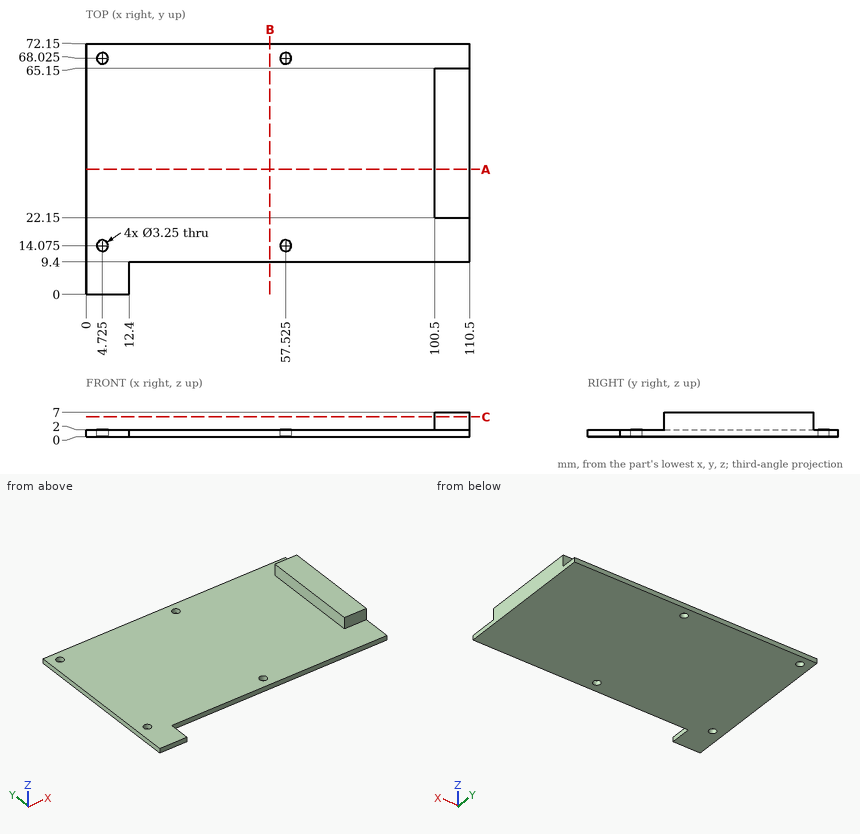
Study the drawing (mm; zero at the part's minimum x, y, z) and answer. Coordinates: 2 decimals unless noted, no trailing zeros. Write each loop counter-clockwise with the first axis right and the second up, starting at its lowest first coordinate (ties: lowest second). Pieces come first, ordered by that corner, then holes. Notation, with made-up numbers: (-18.5, 29.25) - (23.5, 29.25) arc R17 ccw to (23.5, 61.25) - close; hole circle Ø7 at (67, -9). An arc over 180 degrees is marked (long way). Return JSON: item names as keys, results as strings. Group by question number.
1. Given pin 1 (3 mm diameter, centred on x = 4.725, y = 68.025, fed in from -Z); pin 2 (4 mm diameter, centred on y = 49.5, z = 5.5, fed in from -X); pin 3 (0.6 mm diameter, centred on x = 60.5, z = 0.5, fed in from -Y); pin 4 (2.5 mm diameter, centred on x = 106.5, z = 4.5, fed in from +Y), each flat-ended and moving along its own axis, determine where each tip first touches the part or whether it passes through.
2. Straight lines are drawn through the part: L1, parallel to Z at x = 93, y = 48.5; L2, parallel to X at y = 55, z = 4; L3, parallel to Y at x = 97.5, z = 1.75. For each, find the intervals that lie inside material, in ascending order.
3. A cutting plane is placed at A-A, the plane y = 36. Determine the outline of the cut face in (x, z), plus the area to 3 significant figures.
4. A cutting plane is placed at B-B, the plane x = 53. Determine the outline of the cut face in (y, z), plus the area to 4 significant figures.
5. A cutting plane is placed at C-C, the plane z = 5.75. Determine the outline of the cut face in (x, y).
Ans:
{
 "1": {"pin 1": "through", "pin 2": "x = 100.5", "pin 3": "y = 9.4", "pin 4": "y = 65.15"},
 "2": {"L1": "0 to 2", "L2": "100.5 to 110.5", "L3": "9.4 to 72.15"},
 "3": {"outline": "(0, 0) - (110.5, 0) - (110.5, 7) - (100.5, 7) - (100.5, 2) - (0, 2) - close", "area": "271 mm²"},
 "4": {"outline": "(9.4, 0) - (72.15, 0) - (72.15, 2) - (9.4, 2) - close", "area": "125.5 mm²"},
 "5": {"outline": "(100.5, 22.15) - (110.5, 22.15) - (110.5, 65.15) - (100.5, 65.15) - close"}
}
